Answer from the drawing. Dimensions are ordinates in mm from the lowest x, y and z of the part. Give positions to 0.01 mm unless a question says otherwise; leave off trailing zeros. Loops run counter-clockwise (first coordinate to the right, second up) from the corner with the lowest first, then second, coordinate; pieces in that order, holes last. Notation, with made-up numbers: (-2.5, 22.25) - (34.5, 22.25) arc R27 ccw to (34.5, 61.25) - close; hole circle Ø1 at (12, 73.5). An arc over 180 degrees is marked (long way). Answer as CSV lines item,"result". Start each with the question number.
1) A cutting plane is placed at B-B (z = 10.5). Determine the outline of the cut face in (x, y) (1 decimal).
2) A cutting plane is placed at D-D (y = 9.25). Determine the outline of the cut face in (x, z).
3) For a pull along X with two mould halves and no side action, classify the marked faces 1, 2, 3 and 4 as pulls with the +X half, pulls with the -X half, needs draft (parallel to the pull), parting line crosses it, or undercut.
4) Flat-ended cylindrical pins translate along their axes: pin 1 (4 mm diameter, centred on y = 18, z = 11, fed in from -X); pin 2 (4 mm diameter, centred on x = 18, y = 19, fed in from +Z). Find the tip coordinate at first contact, or state that the pin passes through.
5) A cutting plane is placed at C-C (x = 17.4). Determine the outline of the cut face in (y, z).
6) Find the intervals of material crossed by line 1 along X through (y, z) = (12.75, 17.4); line 2 along Z through (x, y) = (17.4, 8.5); line 3 along X through (y, z) = (4.5, 11), in increasing order.
7) A cutting plane is placed at A-A (z = 17.4). Determine the outline of the cut face in (x, y).
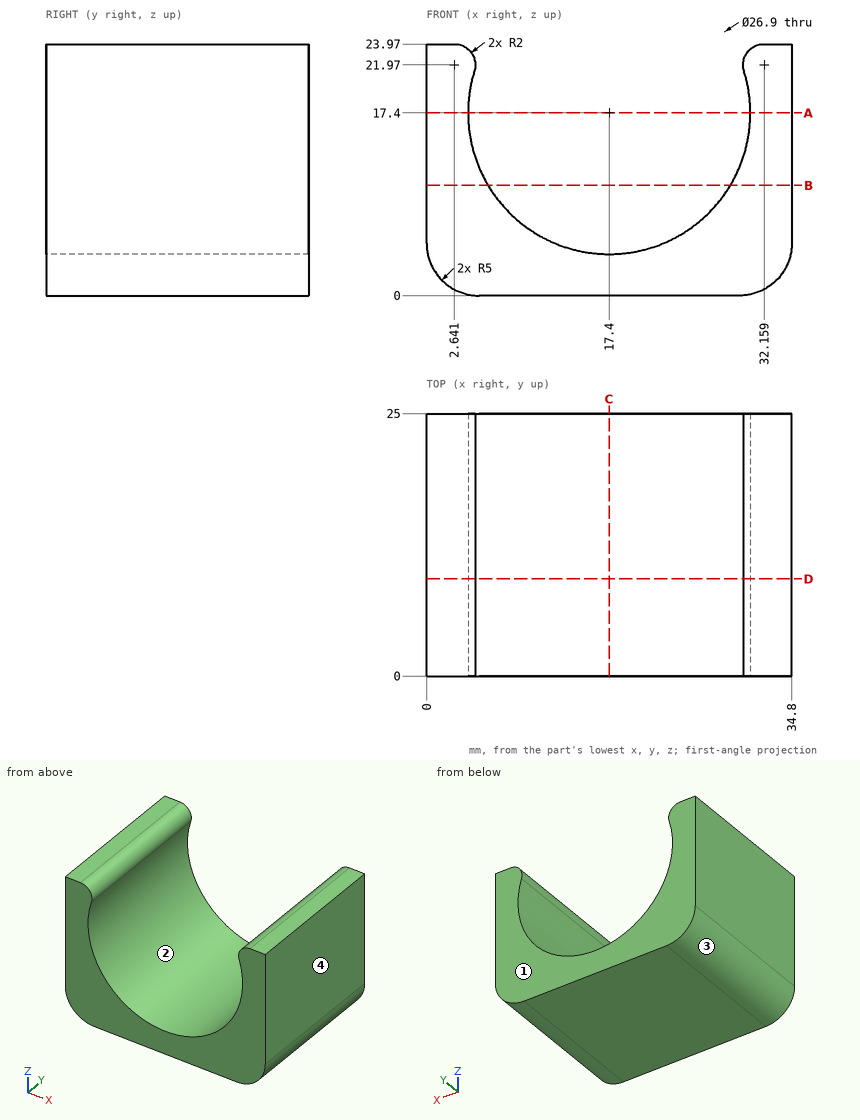
Ans:
1,outline,"(0, 0) - (5.9, 0) - (5.9, 25) - (0, 25) - close; (28.9, 0) - (34.8, 0) - (34.8, 25) - (28.9, 25) - close"
2,outline,"(0, 5) arc R5 ccw to (5, 0) - (29.8, 0) arc R5 ccw to (34.8, 5) - (34.8, 23.97) - (32.16, 23.97) arc R2 ccw to (30.25, 21.38) arc R13.45 cw (long way) to (4.55, 21.38) arc R2 ccw to (2.64, 23.97) - (0, 23.97) - close"
3,face 1,"needs draft"
3,face 2,"undercut"
3,face 3,"pulls with the -X half"
3,face 4,"pulls with the +X half"
4,pin 1,"x = 0"
4,pin 2,"z = 4.2"
5,outline,"(0, 0) - (25, 0) - (25, 3.95) - (0, 3.95) - close"
6,line 1,"0 to 3.95, 30.85 to 34.8"
6,line 2,"0 to 3.95"
6,line 3,"0 to 5.57, 29.23 to 34.8"
7,outline,"(0, 0) - (3.95, 0) - (3.95, 25) - (0, 25) - close; (30.85, 0) - (34.8, 0) - (34.8, 25) - (30.85, 25) - close"
